Geometry check sheet. Reference: the model listing, model coordinates, mm. A direction names the side the tool comes from. Give positions to 0.01 mm unless a question says otherwise; leave off trailing zeros. Loops run counter-clockwise (first coordinate to the right, second up) from the corner with the lowest first, then second, coordinate; pieces in that order, holes last.
1. Cross-section at A-A, the plane x = 0. Record the cut outline in (y, z) (3 decimals), plus the area to 3 significant figures.
2. Cross-section at D-D, the plane x = 19. Record the cut outline in (y, z) (3 decimals), plus the area to 3 significant figures.
3. Cross-section at B-B, the plane z = 0. Record the cut outline in (x, y) (3 decimals).
4. Tool access check on faces 1 (the cylindrical face through (37.46, 2.45, 27.63)), 2 (the flat face through (32, -40.333, 7)), 3 (the cylindrical face through (-23.05, -16.19, -41.56)), 4 (the cylindrical face through (44.35, 2.45, -14.16)), 5 (the flat face through (21.68, -13.44, -30.81)). Record the directions out of +Z, -Z, +X, -X, +Y, -Y that give a thin tool (end or side, any length) a straight path to the whole face; none if there is none.
5. Release check for a two-part mould opening along X. For faces 6 (the cylindrical face through (-23.05, -16.19, 41.56)), 7 (the flat face through (9, -35.6, 37.9)), 8 (the flat face through (22.12, -13.44, 30.49)) record: +X half, -X half, draft (parallel to the pull), parting line (faces both ways), or undercut.
6. Go/stop test with flat-tipped pins: pin 1 Ø1.7 at (x, y) = (39.5, -22.5) entering from -Z; pin 2 Ø1.2 at (x, y) = (43.5, -14) entering from +Z; pin 3 Ø6 at (x, y) = (18, -11) entering from -Z. Record where each tip stops, or that it passes through.
7. Material ranges on L1, parallel to Z at x = 0, y = -29 (3 decimals); L2, parallel to Z at x = 14, y = -8; L3, parallel to Y at x = 41, z = 8 (3 decimals), recorded low to high.
8. Cross-section at C-C, the plane y = -23. State how many separate pieces and enclosed holes the cut face has, plus the area to 3 significant figures.
from build123d import *

# Parameters (mm, degrees)
SKETCH1_R           = 48.26
SKETCH1_R_2         = 32.385
BOSS_EXTRUDE1_DEPTH = 47.625
CUT_EXTRUDE2_START  = -43.50766
CUT_EXTRUDE2_DEPTH  = 43.50766
SKETCH3_W           = 4.572
SKETCH3_H           = 29.845
CUT_EXTRUDE3_DEPTH  = 9.525
SKETCH4_W           = 29.845
SKETCH4_H           = 43.50766
CUT_EXTRUDE4_DEPTH  = 26.400930862
SKETCH5_W           = 29.845
SKETCH5_H           = 43.50766
CUT_EXTRUDE5_DEPTH  = 7.273566766
SKETCH6_W           = 29.845
SKETCH6_H           = 43.50766
CUT_EXTRUDE6_DEPTH  = 26.400930862
CUT_EXTRUDE7_DEPTH  = 48.625
FILLET1_R           = 2.54
FILLET2_R           = 2.54


with BuildPart() as part:
    # Sketch1 → Boss-Extrude1 (new body)
    with BuildSketch(Plane(origin=(0, -40.33266, 0), x_dir=(1, 0, 0), z_dir=(0, 1, 0))):
        Circle(SKETCH1_R)
        Circle(SKETCH1_R_2, mode=Mode.SUBTRACT)
    extrude(amount=BOSS_EXTRUDE1_DEPTH)

    # Sketch2 → Cut-Extrude2 (cut)
    with BuildSketch(Plane.XZ.offset(40.33266).offset(CUT_EXTRUDE2_START)):
        Polygon((40.557916835, -22.48144085), (8.658940442, -45.556366746), (6.128142118, -42.057769336), (37.668433234, -19.242307445), (37.668433234, 19.242307445), (6.128142118, 42.057769336), (8.658940442, 45.556366746), (40.557916835, 22.48144085), (38.535041098, 19.685), (41.986433234, 19.685), (41.986433234, -19.685), (38.535041098, -19.685), align=None)
    extrude(amount=CUT_EXTRUDE2_DEPTH, mode=Mode.SUBTRACT)

    # Sketch3 → Cut-Extrude3 (cut)
    with BuildSketch(Plane(origin=(0, -40.33266, 0), x_dir=(1, 0, 0), z_dir=(0, 1, 0))):
        Polygon((10.731241711, 40.295446893), (8.051572897, 36.591049635), (32.233055001, 19.098767101), (34.912723815, 22.803164359), align=None)
        with Locations((36.652433234, 0)):
            Rectangle(SKETCH3_W, SKETCH3_H)
        Polygon((32.233055001, -19.098767101), (8.051572897, -36.591049635), (10.731241711, -40.295446893), (34.912723815, -22.803164359), align=None)
    extrude(amount=CUT_EXTRUDE3_DEPTH, mode=Mode.SUBTRACT)

    # Sketch4 → Cut-Extrude4 (cut, through all)
    with BuildSketch(Plane(origin=(24.608428639, 0, -34.018903798), x_dir=(0.810235621, 0, 0.58610429), z_dir=(-0.58610429, 0, 0.810235621))):
        with Locations((0, -18.57883)):
            Rectangle(SKETCH4_W, SKETCH4_H)
    extrude(amount=-CUT_EXTRUDE4_DEPTH, mode=Mode.SUBTRACT)

    # Sketch5 → Cut-Extrude5 (cut, through all)
    with BuildSketch(Plane.ZY.offset(-41.986433234)):
        with Locations((0, -18.57883)):
            Rectangle(SKETCH5_W, SKETCH5_H)
    extrude(amount=-CUT_EXTRUDE5_DEPTH, mode=Mode.SUBTRACT)

    # Sketch6 → Cut-Extrude6 (cut, through all)
    with BuildSketch(Plane(origin=(24.608428639, 0, 34.018903798), x_dir=(-0.810235621, 0, 0.58610429), z_dir=(-0.58610429, 0, -0.810235621))):
        with Locations((0, -18.57883)):
            Rectangle(SKETCH6_W, SKETCH6_H)
    extrude(amount=-CUT_EXTRUDE6_DEPTH, mode=Mode.SUBTRACT)

    # Sketch7 → Cut-Extrude7 (cut, through all)
    with BuildSketch(Plane.XZ.offset(40.33266)):
        with BuildLine():
            Line((0, 0), (-24.13, 41.794385987))
            ThreePointArc((-24.13, 41.794385987), (-48.26, 0), (-24.13, -41.794385987))
            Line((-24.13, -41.794385987), (0, 0))
        make_face()
    extrude(amount=-CUT_EXTRUDE7_DEPTH, mode=Mode.SUBTRACT)

    # Fillet1
    fillet1_edges = [part.edges().sort_by_distance(p)[0] for p in [
        (-16.1925, -16.52016, 28.046232702),
        (-16.1925, -16.52016, -28.046232702),
        (-24.13, -16.52016, -41.794385987),
        (-24.13, -16.52016, 41.794385987),
    ]]
    fillet(fillet1_edges, radius=FILLET1_R)

    # Fillet2
    fillet2_edges = [part.edges().sort_by_distance(p)[0] for p in [
        (13.663087314, 3.175, -44.348455518),
        (37.844569418, 3.175, -26.856172984),
        (43.940692479, 3.175, -14.9225),
        (43.940692479, 3.175, 14.9225),
        (37.844569418, 3.175, 26.856172984),
        (13.663087314, 3.175, 44.348455518),
    ]]
    fillet(fillet2_edges, radius=FILLET2_R)


solid = part.part
Result:
1. outline: (-40.333, -48.26) - (7.292, -48.26) - (7.292, -32.385) - (-40.333, -32.385) - close; (-40.333, 32.385) - (7.292, 32.385) - (7.292, 48.26) - (-40.333, 48.26) - close
1. area: 1,510 mm2
2. outline: (-40.333, -28.671) - (-30.808, -28.671) - (-30.808, -32.747) - (3.175, -32.747) - (3.175, -44.362) - (7.292, -44.362) - (7.292, -26.226) - (-40.333, -26.226) - close; (-40.333, 26.226) - (7.292, 26.226) - (7.292, 44.362) - (3.175, 44.362) - (3.175, 32.747) - (-30.808, 32.747) - (-30.808, 28.671) - (-40.333, 28.671) - close
2. area: 639 mm2
3. outline: (32.385, -40.333) - (34.366, -40.333) - (34.366, -30.808) - (37.668, -30.808) - (37.668, 3.175) - (48.26, 3.175) - (48.26, 7.292) - (32.385, 7.292) - close
4. face 1: +Z, -Y
4. face 2: +Z, -Z, +X, -X, -Y
4. face 3: -X, +Y, -Y
4. face 4: +X, -Y
4. face 5: -Y
5. face 6: -X half
5. face 7: +X half
5. face 8: undercut
6. pin 1: stops at z = -28.44
6. pin 2: stops at z = 22.1
6. pin 3: stops at z = -35.64
7. L1: z = -48.26 to -32.385, 32.385 to 48.26
7. L2: z = -46.18 to -44.81, -36.36 to -29.2, 29.2 to 36.36, 44.81 to 46.18
7. L3: y = 3.175 to 7.292
8. separate pieces: 3
8. enclosed holes: 0
8. area: 1,670 mm2
